Work out the finished part from the listing and answer in its coordinate system (mm). A direction names the side the tool comes from. Coordinates: 2 decimals unless noted, no trailing zeros. Write each loop counter-clockwise with the first axis right and the second up, starting at its lowest first coordinate (ties: lowest second). Pieces come first, ordered by that corner, then holes. Notation, with made-up numbers: (-5, -18.5) - (38, -18.5) arc R17 cw to (38, -9.5) - close; hole circle Ø2 at (16, 16.25). An arc over 180 degrees is marked (long way). One line per item, written item: value.
```python
from build123d import *

# Parameters (mm, degrees)
F1_DEPTH = 19.05


with BuildPart() as f1:
    # F0 (on Front) → F1 (new body, symmetric)
    with BuildSketch(Plane.XZ):
        Polygon((27.015501, 121.247835), (38.846832, 121.247835), (38.969941, 133.192345), (-5.387122, 133.192345), (-5.387122, 121.247835), align=None)
        Polygon((-9.170749, 44.403642), (0, 59.079908), (38.846832, 121.247835), (27.015501, 121.247835), (-43.718703, 8.049446), (-43.718703, -10.884642), align=None)
        Polygon((0, -85.755453), (0, 59.079908), (-9.170749, 44.403642), (-9.170749, -85.624769), align=None)
    extrude(amount=F1_DEPTH, both=True)


solid = f1.part
```
Item 1: Given pin 1 (4 mm diameter, centred on x = 11, y = -9, fed in from -Z); pin 2 (10 mm diameter, centred on x = -11.5, z = -13, fed in from +Y); pin 3 (10 mm diameter, centred on y = 9, z = 41.5, fed in from +X); pin 4 (4 mm diameter, centred on x = -25.5, y = 15, fed in from +Z), each flat-ended and moving along its own axis, determine where each tip first touches the part or whether it passes through.
Evaluation:
pin 1: stops at z = 73.48
pin 2: stops at y = 19.05
pin 3: stops at x = 0
pin 4: stops at z = 40.41
Item 2: Section B-B, the plane z = 16 is taken. Determine the outline of the cut face in (x, y).
Evaluation:
outline: (-38.75, -19.05) - (-26.92, -19.05) - (-26.92, 19.05) - (-38.75, 19.05) - close; (-9.17, -19.05) - (0, -19.05) - (0, 19.05) - (-9.17, 19.05) - close
Item 3: Determine the mould class of faces 1 (the face through (-9.171, 0, -20)), 2 (the face through (19.15, -0.27, 89.73)), 3 (the face through (-7.856, -0.267, 65.441)) for opening direction X: +X half, -X half, draft (parallel to the pull), parting line (faces both ways), or undercut.
Evaluation:
face 1: undercut
face 2: +X half
face 3: -X half
Item 4: Section A-A, the plane x = -2.5 is taken. Determine the outline of the cut face in (y, z), then the cut area to 3 significant figures.
Evaluation:
outline: (-19.05, -85.72) - (19.05, -85.72) - (19.05, 74.01) - (-19.05, 74.01) - close; (-19.05, 121.25) - (19.05, 121.25) - (19.05, 133.19) - (-19.05, 133.19) - close
area: 6,540 mm2
Item 5: Section C-C, the plane y = 2.5 is taken. Determine the outline of the cut face in (x, z), then the cut area to 3 significant figures.
Evaluation:
outline: (-43.72, -10.88) - (-9.17, 44.4) - (-9.17, -85.62) - (0, -85.76) - (0, 59.08) - (38.85, 121.25) - (38.97, 133.19) - (-5.39, 133.19) - (-5.39, 121.25) - (27.02, 121.25) - (-43.72, 8.05) - close
area: 3,240 mm2
Item 6: Section D-D, the plane z = -61 is taken. Determine the outline of the cut face in (x, y), then the cut area to 3 significant figures.
Evaluation:
outline: (-9.17, -19.05) - (0, -19.05) - (0, 19.05) - (-9.17, 19.05) - close
area: 349 mm2
Item 7: Consider probe 1 along X at (y, z) = (0.5, -38.5); probe 2 along Z at (x, y) = (8, -17); probe 3 along Z at (x, y) = (3, 3) (3 decimals). Determine where each line is inside the solid, lowest interval first.
Evaluation:
probe 1: x = -9.17 to 0
probe 2: z = 71.88 to 90.82, 121.25 to 133.19
probe 3: z = 63.881 to 82.815, 121.248 to 133.192
Item 8: Which of the six approach directions +Z, -Z, +X, -X, +Y, -Y give full straight-line access (tool end or side, diameter ignored) to faces 4 (the face through (-3, -19.05, 40)), 5 (the face through (-26.69, -0.27, 16.37)), 6 (the face through (-5.387, 0, 127)), 7 (the face through (11, 0, 121.248)), 8 (the face through (0, 0, -14))?
Evaluation:
face 4: +Z, -Z, +X, -X, -Y
face 5: -Z, +Y, -Y
face 6: +Z, -X, +Y, -Y
face 7: -X, +Y, -Y
face 8: -Z, +X, +Y, -Y
